Autodesk Inventor part; units mm, degrees
ref_plane "YZ Plane" through (0, 0, 0) normal (1, 0, 0) x (0, 1, 0)
ref_plane "XZ Plane" through (0, 0, 0) normal (0, 1, 0) x (-1, 0, 0)
ref_plane "XY Plane" through (0, 0, 0) normal (0, 0, 1) x (1, 0, 0)
sketch "Sketch1" plane through (0, 0, 0) normal (0, 0, 1) x (1, 0, 0)
  line L0 (0, 0) -> (-75, 0)
  line L1 (-75, 0) -> (-75, 95)
  line L2 (-75, 95) -> (0, 95)
  line L3 (0, 95) -> (0, 0)
  line L4 (-65, 85) -> (-10, 85)
  line L5 (-10, 85) -> (-10, 10)
  line L6 (-10, 10) -> (-65, 10)
  line L7 (-65, 10) -> (-65, 85)
  dimension "d0" = 75
  dimension "d1" = 95
  dimension "d10" = 55
  dimension "d11" = 75
extrude "Extrusion3" add sketch "Sketch1" along normal blind 10
sketch "Sketch2" plane through (-75, 95, 0) normal (0, 1, 0) x (1, 0, 0)
  line L0 (1, -1) -> (11.6, -1)
  line L1 (11.6, -1) -> (11.6, -6.6)
  line L2 (11.6, -6.6) -> (1, -6.6)
  line L3 (1, -6.6) -> (1, -1)
  line L4 (74, -1) -> (63.4, -1)
  line L5 (63.4, -1) -> (63.4, -6.6)
  line L6 (63.4, -6.6) -> (74, -6.6)
  line L7 (74, -6.6) -> (74, -1)
  point P0 (75, 0)
  dimension "d14" = 10.6
  dimension "d15" = 5.6
  dimension "d16" = 10.6
  dimension "d17" = 5.6
extrude "Extrusion4" cut sketch "Sketch2" against normal blind 5
sketch "Sketch3" plane through (-75, 0, 0) normal (0, -1, 0) x (1, 0, 0)
  line L0 (1, 1) -> (11.6, 1)
  line L1 (11.6, 1) -> (11.6, 6.6)
  line L2 (11.6, 6.6) -> (1, 6.6)
  line L3 (1, 6.6) -> (1, 1)
  line L4 (63.4, 6.6) -> (63.4, 1)
  line L5 (74, 1) -> (63.4, 1)
  line L6 (63.4, 1) -> (63.4, 6.6)
  line L7 (63.4, 6.6) -> (74, 6.6)
  line L8 (74, 6.6) -> (74, 1)
  point P0 (75, 0)
  point P1 (63.4, 1)
  dimension "d20" = 10.6
  dimension "d21" = 5.6
  dimension "d22" = 10.6
  dimension "d23" = 5.6
extrude "Extrusion5" cut sketch "Sketch3" against normal blind 5
properties part number "Shoulder_Cube_TestFit_V1"
Check sheet for the modelled part. Datum: model origin and axes. Units: mm. A direction names the side the tool comes from. Round coordinates to 2 decimals unless told otherwise and drop trailing zeros. Loops run counter-clockwise (first coordinate to the right, second up) from the corner with the lowest first, then second, coordinate; pieces in that order, holes last. Notation, with made-up numbers: (-38.5, 42.5) - (-17.5, 42.5) arc R27 cw to (-17.5, 81.5) - close; hole circle Ø1 at (28, 45). An arc over 180 degrees is marked (long way). Write item = value, one per line. Start each with the question number.
Q1. Section check A-A (y = 30). Record the boundary of the cut face in (x, z).
Q2. Depth check by flat-ended pin: P1, Ø3, axis at x = -8.5, z = 3, coming from the +Y side. Enter the tip coordinate at first touch or a pass-through.
Q3. Section check C-C (x = -25). Record the boundary of the cut face in (y, z).
Q4. Access from +Z, -Z, +X, -X, +Y, -Y to the whole of each face (thin tool, end or side, straight path). Record for faces 1 (the face through (-6, 2, 1)), 2 (the face through (-65, 47, 5)), 3 (the face through (-11.6, 93, 4)).
Q5. Thickness scan on L1, parallel to X at y = 77, z = 1; L2, parallel to Y at x = -25, z = 9. Record the ranges inside material, lowest first.
Q6. Release check for a two-part mould opening along Z. For faces 4 (the face through (-69, 90, 4)), 5 (the face through (-69, 93, 6.6)), 6 (the face through (-37, 0, 5)), 7 (the face through (-5, 48, 0)) record: pulls with the +Z half, pulls with the -Z half, needs draft (parallel to the pull), parting line crosses it, or undercut.
Q7. Section check B-B (z = 4.25). Record the boundary of the cut face in (x, y), plus the area to 3 significant figures.
Derived:
q1.outline = (-75, 0) - (-65, 0) - (-65, 10) - (-75, 10) - close; (-10, 0) - (0, 0) - (0, 10) - (-10, 10) - close
q2.P1 = 90
q3.outline = (0, 0) - (10, 0) - (10, 10) - (0, 10) - close; (85, 0) - (95, 0) - (95, 10) - (85, 10) - close
q4.face_1 = -Y
q4.face_2 = +Z, -Z
q4.face_3 = +Y
q5.L1 = -75 to -65, -10 to 0
q5.L2 = 0 to 10, 85 to 95
q6.face_4 = undercut
q6.face_5 = undercut
q6.face_6 = needs draft
q6.face_7 = pulls with the -Z half
q7.outline = (-75, 0) - (-74, 0) - (-74, 5) - (-63.4, 5) - (-63.4, 0) - (-11.6, 0) - (-11.6, 5) - (-1, 5) - (-1, 0) - (0, 0) - (0, 95) - (-1, 95) - (-1, 90) - (-11.6, 90) - (-11.6, 95) - (-63.4, 95) - (-63.4, 90) - (-74, 90) - (-74, 95) - (-75, 95) - close; hole (-65, 10) - (-10, 10) - (-10, 85) - (-65, 85) - close
q7.area = 2,790 mm^2
